```python
from build123d import *

# Parameters (mm, degrees)
BOSS_EXTRUDE1_DEPTH = 40
BOSS_EXTRUDE2_DEPTH = 3
LPATTERN1_COUNT     = 2
LPATTERN1_PITCH     = 37
CHAMFER1_SIZE       = 1
BOSS_EXTRUDE5_START = -21
SKETCH6_W           = 10
SKETCH6_H           = 49.445125494
SKETCH6_W_2         = 49.445125494
SKETCH6_H_2         = 10
BOSS_EXTRUDE5_DEPTH = 2


with BuildPart() as part:
    # Sketch2 → Boss-Extrude1 (new body)
    with BuildSketch(Plane.XY):
        Polygon((0, 0), (60, 0), (60, 2), (-2, 2), (-2, -60), (0, -60), align=None)
    extrude(amount=BOSS_EXTRUDE1_DEPTH)

    # Sketch3 → Boss-Extrude2 (add)
    with BuildSketch(Plane.XY.offset(40)):
        Polygon((15, 0), (0, 0), (0, -15), align=None)
    boss_extrude2 = extrude(amount=-BOSS_EXTRUDE2_DEPTH)

    # LPattern1: Boss-Extrude2 ×2
    with Locations(*[(0, 0, -i * LPATTERN1_PITCH) for i in range(1, LPATTERN1_COUNT)]):
        add(boss_extrude2)

    # Chamfer1
    chamfer1_edges = [part.edges().sort_by_distance(p)[0] for p in [
        (0, -60, 20),
        (60, 0, 20),
    ]]
    chamfer(chamfer1_edges, length=CHAMFER1_SIZE)

    # Sketch6 → Boss-Extrude5 (add)
    with BuildSketch(Plane.XY.offset(40).offset(BOSS_EXTRUDE5_START)):
        with Locations((-7, -35.277437253)):
            Rectangle(SKETCH6_W, SKETCH6_H)
        with Locations((35.277437253, 7)):
            Rectangle(SKETCH6_W_2, SKETCH6_H_2)
    extrude(amount=BOSS_EXTRUDE5_DEPTH)


solid = part.part
```
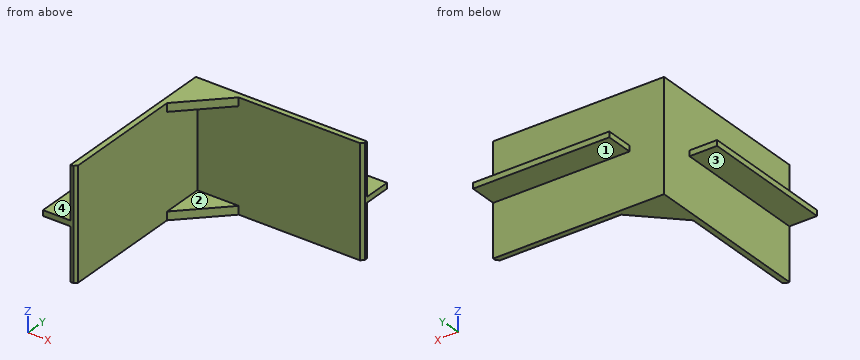
Input: part model. Units: mm. Frame: model coordinates. Face numbers are marked on the shaded views. A direction names the side the tool comes from. Give positions to 0.01 mm unless a question says otherwise; leave off trailing zeros. Order: outer loops, then holes, each group sorted by start corner. A loop starts at its lowest first (then second) coordinate and runs counter-clockwise, first axis right, second up. Notation, with made-up numbers: (62, -32) - (75, -32) arc R36 cw to (75, 4) - close; hole circle Ø11 at (89, -6.75). An arc over 180 degrees is marked (long way). Put each result on its own line as item: value.
Item 1: Section query A-A, the plane x = 4. Return loops of the section in (y, z).
Found:
outline: (-11, 0) - (2, 0) - (2, 40) - (-11, 40) - (-11, 37) - (0, 37) - (0, 3) - (-11, 3) - close
Item 2: Section query C-C, the plane x = -7. Return loops of the section in (y, z).
Found:
outline: (-60, 19) - (-10.55, 19) - (-10.55, 21) - (-60, 21) - close
Item 3: Section query D-D, the plane y = 7.5. Return loops of the section in (x, z).
Found:
outline: (10.55, 19) - (60, 19) - (60, 21) - (10.55, 21) - close
Item 4: Contact query for flat-ended pins moving along their axis: pin 1 (20 mm diameter, centred on y = -38.5, z = 11, fed in from +X); pin 2 (1 mm diameter, centred on x = 44.5, z = 8.5, fed in from +Y); pin 3 (8 mm diameter, centred on x = 27.5, y = 6.5, fed in from -Z); pin 4 (10 mm diameter, centred on x = 10, y = -18, fed in from -Z). Output: stop coordinate, or through.
Found:
pin 1: stops at x = 0
pin 2: stops at y = 2
pin 3: stops at z = 19
pin 4: passes through
Item 5: Access query for the marked faces 1, 2, 3 and 4. Directions: +Z, -Z, +X, -X, +Y, -Y. A direction counts if a zero-diameter tool reaches every point of the face in a straight line with its end or side. Return the directions, or none.
Found:
face 1: -Z, +X, -X, +Y
face 2: +X, -Y
face 3: -Z, -X, +Y, -Y
face 4: +Z, -X, +Y, -Y
Item 6: Ray query, L1, parallel to Y at x = 56.5, z = 9; L2, parallel to Z at x = -2.5, y = -51; L3, parallel to X at y = -50.5, z = 37.5. Return the intervals inside material, ascending. Write a range as from..to.
Found:
L1: y = 0..2
L2: z = 19..21
L3: x = -2..0
Item 7: Section query B-B, the plane y = -51. Return loops of the section in (x, z).
Found:
outline: (-12, 19) - (-2, 19) - (-2, 0) - (0, 0) - (0, 40) - (-2, 40) - (-2, 21) - (-12, 21) - close
